Source: CAD feature listing. Evaluate the final solid. Frame: model axes, mm. A direction names the side the tool comes from. Give positions to 0.01 mm unless a question says otherwise; leave off trailing zeros. Order: outer loops, then holes, each group sorted by start corner. A loop starts at its lowest first (then second) coordinate and runs counter-clockwise, first axis right, second up. Notation, with made-up numbers: (-3.5, 22.25) - (16.5, 22.25) arc R28 cw to (16.5, 61.25) - close; hole circle Ø1 at (68, 30.5). An arc over 180 degrees is marked (long way). Answer as CSV lines item,"result".
```python
from build123d import *

# Parameters (mm, degrees)
BOSS_EXTRUDE1_DEPTH = 9.525
CUT_EXTRUDE1_REACH  = 11.525
SKETCH2_R           = 2.54
SKETCH2_W           = 6.35
SKETCH2_H           = 30


with BuildPart() as part:
    # Sketch1 → Boss-Extrude1 (new body)
    with BuildSketch(Plane(origin=(0, 0, 0), x_dir=(1, 0, 0), z_dir=(0, 1, 0))):
        with BuildLine():
            Line((25.4, 0), (196.85, 0))
            ThreePointArc((196.85, 0), (201.340128061, 1.859871939), (203.2, 6.35))
            Line((203.2, 6.35), (203.2, 247.65))
            ThreePointArc((203.2, 247.65), (201.340128061, 252.140128061), (196.85, 254))
            Line((196.85, 254), (25.4, 254))
            ThreePointArc((25.4, 254), (7.439487758, 246.560512242), (0, 228.6))
            Line((0, 228.6), (0, 25.4))
            ThreePointArc((0, 25.4), (7.439487758, 7.439487758), (25.4, 0))
        make_face()
    extrude(amount=BOSS_EXTRUDE1_DEPTH)

    # Sketch2 → Cut-Extrude1 (cut, up to next)
    with BuildSketch(Plane(origin=(0, 9.525, 0), x_dir=(1, 0, 0), z_dir=(0, 1, 0)), mode=Mode.PRIVATE) as cut_extrude1_sk1:
        with Locations((174.85000082, 40.4)):
            Circle(SKETCH2_R)
    cut_extrude1_tool1 = extrude(cut_extrude1_sk1.sketch, amount=-CUT_EXTRUDE1_REACH, mode=Mode.PRIVATE) & part.part
    add(cut_extrude1_tool1.solids().sort_by_distance((174.850001, 9.525, -40.4))[0], mode=Mode.SUBTRACT)
    # Sketch2 → Cut-Extrude1 (cut, up to next)
    with BuildSketch(Plane(origin=(0, 9.525, 0), x_dir=(1, 0, 0), z_dir=(0, 1, 0)), mode=Mode.PRIVATE) as cut_extrude1_sk2:
        with Locations((183.8500006, 49.39999978)):
            Circle(SKETCH2_R)
    cut_extrude1_tool2 = extrude(cut_extrude1_sk2.sketch, amount=-CUT_EXTRUDE1_REACH, mode=Mode.PRIVATE) & part.part
    add(cut_extrude1_tool2.solids().sort_by_distance((183.850001, 9.525, -49.4))[0], mode=Mode.SUBTRACT)
    # Sketch2 → Cut-Extrude1 (cut, up to next)
    with BuildSketch(Plane(origin=(0, 9.525, 0), x_dir=(1, 0, 0), z_dir=(0, 1, 0)), mode=Mode.PRIVATE) as cut_extrude1_sk3:
        with Locations((183.8500006, 31.40000022)):
            Circle(SKETCH2_R)
    cut_extrude1_tool3 = extrude(cut_extrude1_sk3.sketch, amount=-CUT_EXTRUDE1_REACH, mode=Mode.PRIVATE) & part.part
    add(cut_extrude1_tool3.solids().sort_by_distance((183.850001, 9.525, -31.4))[0], mode=Mode.SUBTRACT)
    # Sketch2 → Cut-Extrude1 (cut, up to next)
    with BuildSketch(Plane(origin=(0, 9.525, 0), x_dir=(1, 0, 0), z_dir=(0, 1, 0)), mode=Mode.PRIVATE) as cut_extrude1_sk4:
        with Locations((174.85000082, 161.05)):
            Circle(SKETCH2_R)
    cut_extrude1_tool4 = extrude(cut_extrude1_sk4.sketch, amount=-CUT_EXTRUDE1_REACH, mode=Mode.PRIVATE) & part.part
    add(cut_extrude1_tool4.solids().sort_by_distance((174.850001, 9.525, -161.05))[0], mode=Mode.SUBTRACT)
    # Sketch2 → Cut-Extrude1 (cut, up to next)
    with BuildSketch(Plane(origin=(0, 9.525, 0), x_dir=(1, 0, 0), z_dir=(0, 1, 0)), mode=Mode.PRIVATE) as cut_extrude1_sk5:
        with Locations((183.8500006, 170.04999978)):
            Circle(SKETCH2_R)
    cut_extrude1_tool5 = extrude(cut_extrude1_sk5.sketch, amount=-CUT_EXTRUDE1_REACH, mode=Mode.PRIVATE) & part.part
    add(cut_extrude1_tool5.solids().sort_by_distance((183.850001, 9.525, -170.05))[0], mode=Mode.SUBTRACT)
    # Sketch2 → Cut-Extrude1 (cut, up to next)
    with BuildSketch(Plane(origin=(0, 9.525, 0), x_dir=(1, 0, 0), z_dir=(0, 1, 0)), mode=Mode.PRIVATE) as cut_extrude1_sk6:
        with Locations((183.8500006, 152.05000022)):
            Circle(SKETCH2_R)
    cut_extrude1_tool6 = extrude(cut_extrude1_sk6.sketch, amount=-CUT_EXTRUDE1_REACH, mode=Mode.PRIVATE) & part.part
    add(cut_extrude1_tool6.solids().sort_by_distance((183.850001, 9.525, -152.05))[0], mode=Mode.SUBTRACT)
    # Sketch2 → Cut-Extrude1 (cut, up to next)
    with BuildSketch(Plane(origin=(0, 9.525, 0), x_dir=(1, 0, 0), z_dir=(0, 1, 0)), mode=Mode.PRIVATE) as cut_extrude1_sk7:
        with Locations((200.025, 40.4)):
            Rectangle(SKETCH2_W, SKETCH2_H)
    cut_extrude1_tool7 = extrude(cut_extrude1_sk7.sketch, amount=-CUT_EXTRUDE1_REACH, mode=Mode.PRIVATE) & part.part
    add(cut_extrude1_tool7.solids().sort_by_distance((200.025, 9.525, -40.4))[0], mode=Mode.SUBTRACT)
    # Sketch2 → Cut-Extrude1 (cut, up to next)
    with BuildSketch(Plane(origin=(0, 9.525, 0), x_dir=(1, 0, 0), z_dir=(0, 1, 0)), mode=Mode.PRIVATE) as cut_extrude1_sk8:
        with Locations((200.025, 161.05)):
            Rectangle(SKETCH2_W, SKETCH2_H)
    cut_extrude1_tool8 = extrude(cut_extrude1_sk8.sketch, amount=-CUT_EXTRUDE1_REACH, mode=Mode.PRIVATE) & part.part
    add(cut_extrude1_tool8.solids().sort_by_distance((200.025, 9.525, -161.05))[0], mode=Mode.SUBTRACT)


solid = part.part
```
(1) Cut plane A-A (y = 2.5). Return loops of the section in (x, z), then the cut area to 3 significant figures.
Completed:
outline,"(0, -228.6) arc R25.4 ccw to (25.4, -254) - (196.85, -254) arc R6.35 ccw to (203.2, -247.65) - (203.2, -176.05) - (196.85, -176.05) - (196.85, -146.05) - (203.2, -146.05) - (203.2, -55.4) - (196.85, -55.4) - (196.85, -25.4) - (203.2, -25.4) - (203.2, -6.35) arc R6.35 ccw to (196.85, 0) - (25.4, 0) arc R25.4 ccw to (0, -25.4) - close; hole circle Ø5.08 at (174.85, -161.05); hole circle Ø5.08 at (174.85, -40.4); hole circle Ø5.08 at (183.85, -170.05); hole circle Ø5.08 at (183.85, -152.05); hole circle Ø5.08 at (183.85, -49.4); hole circle Ø5.08 at (183.85, -31.4)"
area,"50,800 mm²"
(2) Access query for faces 4 (the flat face through (200, 5, -146.05)), 5 (the flat face through (203.2, 5, -16)). Directions: +Z, -Z, +X, -X, +Y, -Y. A direction counts if a zero-diameter tool reaches every point of the face in a straight line with its end or side. Return the directions, or none.
Completed:
face 4,"+X, +Y, -Y"
face 5,"+Z, -Z, +X, +Y, -Y"
(3) Ray query, line 1 (Z direction, x = 174.85, y = 2.25); line 2 (Z direction, x = 183.85, y = 2); line 3 (Z direction, x = 175.5, y = 2). Return the intervals inside material, ascending. Write a range as from..to.
Completed:
line 1,"-254..-163.59, -158.51..-42.94, -37.86..0"
line 2,"-254..-172.59, -167.51..-154.59, -149.51..-51.94, -46.86..-33.94, -28.86..0"
line 3,"-254..-163.51, -158.59..-42.86, -37.94..0"
(4) Mould query, pull axis Z, two halves, no side actions, for faces 1 (the flat face through (203.2, 5, -211)), 2 (the flat face through (200, 5, -55.4)), 3 (the flat face through (110, 5, 0)). Classes: released by +Z, released by -Z, zero draft, split by the parting line, or undercut.
Completed:
face 1,"zero draft"
face 2,"undercut"
face 3,"released by +Z"
(5) Contact query for flat-ended pins moving along their axis: pin 1 (4.5 mm diameter, centred on x = 183.85, z = -170.05, fed in from -Y); pin 2 (3 mm diameter, centred on x = 199.5, y = 4, fed in from +Z) (3 decimals); pin 3 (2 mm diameter, centred on y = 2.5, z = -167, fed in from +X); pin 4 (1.9 mm diameter, centred on x = 200, y = 5, fed in from -Z). Output: stop coordinate, or through.
Completed:
pin 1,"through"
pin 2,"z = -0.105"
pin 3,"x = 196.85"
pin 4,"z = -253.61"
